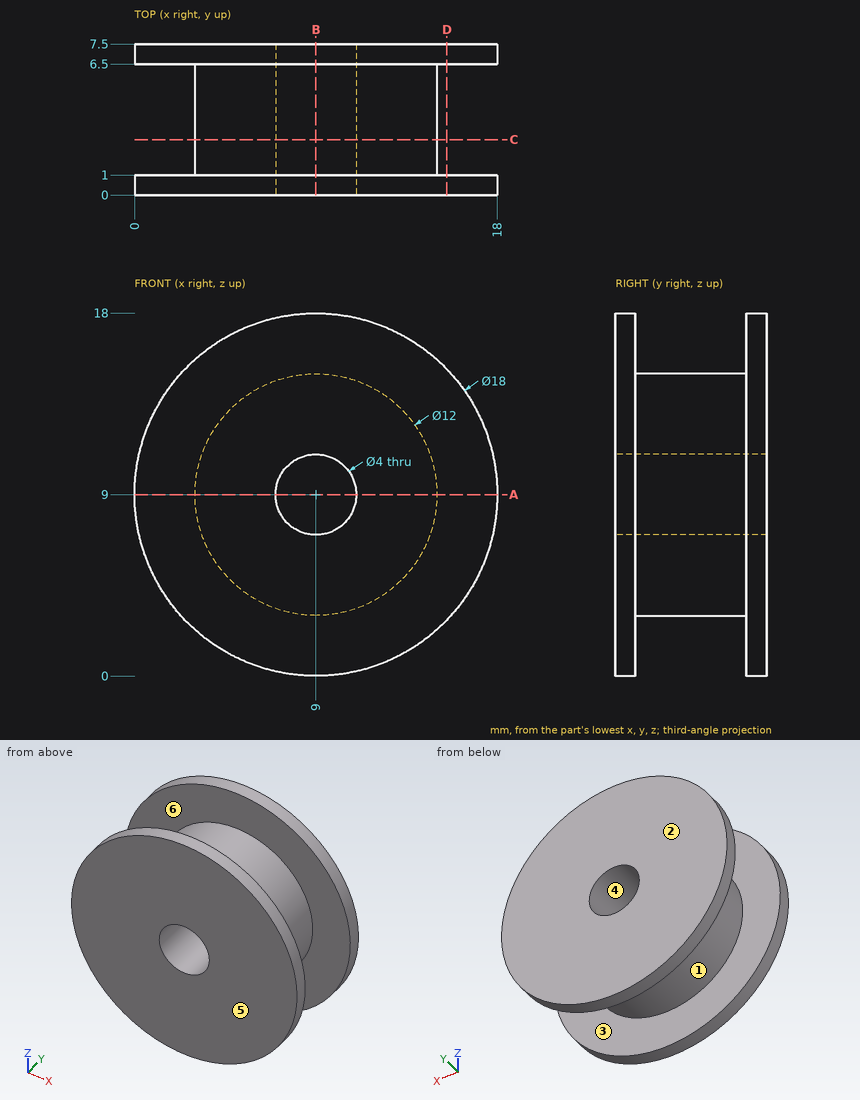
Part print with two shaded views. Sizes in mm from the minimum x, y, z corner. A direction names the side the tool comes from. Round coordinates to 2 decimals unless told otherwise and drop trailing zeros. Order: outer loops, then holes, each group sorted by start corner. A loop starts at its lowest first (then second) coordinate and runs counter-clockwise, first axis right, second up.
(1) Band-saw the part on A-A (z = 9). List the corners of the cut face in (x, y).
(2) Pull direction Y, two halves, no side cores. Call the marked faces 3, 4, 5 and 6: released by +Y, released by -Y, zero draft, split by the parting line, or undercut.
(3) Band-saw the part on B-B (x = 9). List the corners of the cut face in (y, z).
(4) 3-axis set-ups, long thin cutter, end or side, ignore diameter. For the marked faces 1 and 2: which of +Z, -Z, +X, -X, +Y, -Y reach the whole face in a straight line?
(5) Pin check, flat tip, straight feed: pin 1 (4 mm diameter, centred on x = 16, y = 1.5, fed in from +Z). Stop position of the tip, or through.
(6) Band-saw the part on D-D (x = 15.5). List the corners of the cut face in (y, z), then the cut area to 3 significant figures.
(7) Band-saw the part on C-C (y = 2.75). List the corners of the cut face in (x, z), then the cut area to 3 significant figures.
(8) Drill centre lines: line 1 (X direction, y = 5.5, z = 9); line 2 (Y direction, x = 9.75, z = 17); line 3 (X direction, y = 7, z = 7.75). Where is each one in solid material? Low to high.
Verdict:
1. outline: (0, 0) - (7, 0) - (7, 7.5) - (0, 7.5) - (0, 6.5) - (3, 6.5) - (3, 1) - (0, 1) - close; (11, 0) - (18, 0) - (18, 1) - (15, 1) - (15, 6.5) - (18, 6.5) - (18, 7.5) - (11, 7.5) - close
2. face 3: undercut
2. face 4: zero draft
2. face 5: released by -Y
2. face 6: undercut
3. outline: (0, 0) - (1, 0) - (1, 3) - (6.5, 3) - (6.5, 0) - (7.5, 0) - (7.5, 7) - (0, 7) - close; (0, 11) - (7.5, 11) - (7.5, 18) - (6.5, 18) - (6.5, 15) - (1, 15) - (1, 18) - (0, 18) - close
4. face 1: none
4. face 2: +Z, -Z, +X, -X, +Y
5. pin 1: stops at z = 16.44
6. outline: (0, 2.78) - (1, 2.78) - (1, 15.22) - (0, 15.22) - close; (6.5, 2.78) - (7.5, 2.78) - (7.5, 15.22) - (6.5, 15.22) - close
6. area: 24.9 mm2
7. outline: circle Ø12 at (9, 9); hole circle Ø4 at (9, 9)
7. area: 101 mm2
8. line 1: x = 3 to 7, 11 to 15
8. line 2: y = 0 to 1, 6.5 to 7.5
8. line 3: x = 0.09 to 7.44, 10.56 to 17.91
